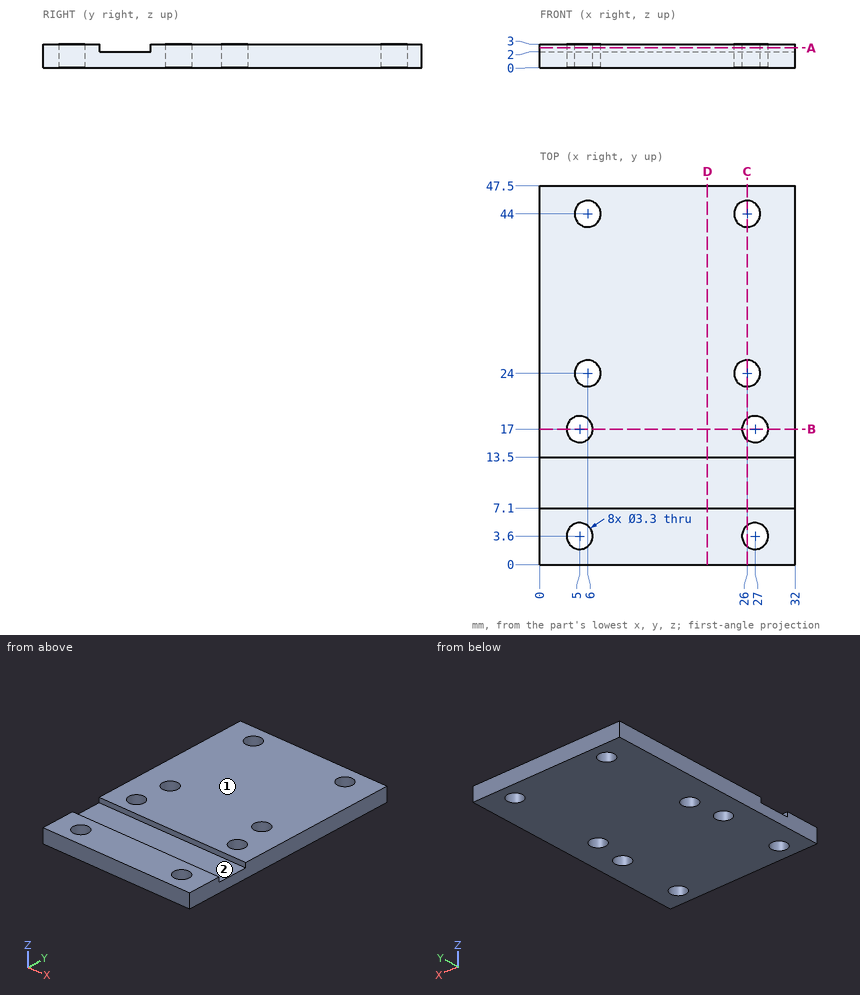
Design review of the part shown in the three views and the two pictorial views. Dimensions are in mm from the part's minimum x, y and z. Coordinates: 2 decimals unless noted, no trailing zeros. Loops run counter-clockwise (first coordinate to the right, second up) from the corner with the lowest first, then second, coordinate; pieces in that order, holes last. Notation, with made-up numbers: (-18.75, -4.75) -> (24.25, -4.75) arc R27 ccw to (24.25, 34.25) -> close; hole circle Ø7 at (-16, -20.75). An arc over 180 degrees is marked (long way). Answer as CSV lines item,"result".
Item 1: Take a section at B-B, the plane y = 17. State the section outline as (x, z) points, and give its area (3 significant figures).
Results below:
outline,"(0, 0) -> (3.35, 0) -> (3.35, 3) -> (0, 3) -> close; (6.65, 0) -> (25.35, 0) -> (25.35, 3) -> (6.65, 3) -> close; (28.65, 0) -> (32, 0) -> (32, 3) -> (28.65, 3) -> close"
area,"76.2 mm2"
Item 2: Take a section at C-C, the plane x = 26. State the section outline as (y, z) points.
Results below:
outline,"(0, 0) -> (2.29, 0) -> (2.29, 3) -> (0, 3) -> close; (4.91, 0) -> (15.69, 0) -> (15.69, 3) -> (13.5, 3) -> (13.5, 2) -> (7.1, 2) -> (7.1, 3) -> (4.91, 3) -> close; (18.31, 0) -> (22.35, 0) -> (22.35, 3) -> (18.31, 3) -> close; (25.65, 0) -> (42.35, 0) -> (42.35, 3) -> (25.65, 3) -> close; (45.65, 0) -> (47.5, 0) -> (47.5, 3) -> (45.65, 3) -> close"
Item 3: For L1, parallel to X at y = 17.5, z = 0.7; L2, parallel to X at y = 18, z = 0.7; L3, parallel to Y at x = 26, z = 1.9, list the stretches that pass through material, from the lowest coordinate up.
Results below:
L1,"x = 0 to 3.43, 6.57 to 25.43, 28.57 to 32"
L2,"x = 0 to 3.69, 6.31 to 25.69, 28.31 to 32"
L3,"y = 0 to 2.29, 4.91 to 15.69, 18.31 to 22.35, 25.65 to 42.35, 45.65 to 47.5"
Item 4: Insertion check: pin 1 (2 mm diameter, centred on x = 26, y = 24, fed in from -Z). The pin has a flat end and moves straight along its axis. Give the tip position at first contact, or say it passes through.
Results below:
pin 1,"passes through"
Item 5: Take a section at A-A, the plane z = 2.5. Count the separate pieces of the cut face and the enclosed holes in it, and give its area (3 significant figures).
Results below:
separate pieces,"2"
enclosed holes,"8"
area,"1,250 mm2"
Item 6: Draft analysis for pull direction Y (two halves, no side actions). For the marked faces 1 and 2, state which applies: +Y half, -Y half, draft (parallel to the pull), parting line (faces both ways), or undercut.
Results below:
face 1,"draft"
face 2,"undercut"
Item 7: Take a section at D-D, the plane x = 21. State the section outline as (y, z) points, and give its area (3 significant figures).
Results below:
outline,"(0, 0) -> (47.5, 0) -> (47.5, 3) -> (13.5, 3) -> (13.5, 2) -> (7.1, 2) -> (7.1, 3) -> (0, 3) -> close"
area,"136 mm2"
